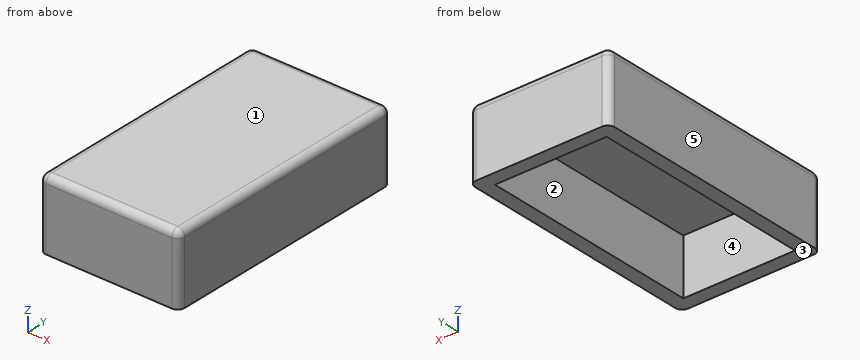
Autodesk Inventor part; units mm, degrees
ref_plane "YZ Plane" through (0, 0, 0) normal (1, 0, 0) x (0, 1, 0)
ref_plane "XZ Plane" through (0, 0, 0) normal (0, 1, 0) x (-1, 0, 0)
ref_plane "XY Plane" through (0, 0, 0) normal (0, 0, 1) x (1, 0, 0)
sketch "Sketch1" plane through (0, 0, 0) normal (0, 0, 1) x (1, 0, 0)
  line L0 (-25.4, -50.8) -> (25.4, -50.8)
  line L1 (25.4, -50.8) -> (25.4, 50.8)
  line L2 (25.4, 50.8) -> (-25.4, 50.8)
  line L3 (-25.4, 50.8) -> (-25.4, -50.8)
  line L4 (-25.4, -50.8) -> (25.4, 50.8) construction
  line L5 (25.4, -50.8) -> (-25.4, 50.8) construction
  point P0 (0, 0)
  dimension "d0" = 50.8
  dimension "d1" = 101.6
extrude "Extrusion1" add sketch "Sketch1" along normal blind 6.35
sketch "Sketch2" plane through (25.4, -50.8, 0) normal (1, 0, 0) x (0, 0, -1)
  line L0 (-6.35, 0) -> (-6.35, 101.6)
  line L1 (-6.35, 101.6) -> (0, 101.6)
  line L2 (0, 101.6) -> (0, 0)
  line L3 (0, 0) -> (-6.35, 0)
  line L4 (-6.35, 0) -> (-6.35, 101.6)
  point P0 (0, 50.8)
extrude "Extrusion2" add sketch "Sketch2" along normal blind 6.35
sketch "Sketch3" plane through (-25.4, -50.8, 0) normal (-1, 0, 0) x (0, 0, 1)
  point P0 (0, 50.8)
sketch "Sketch4" plane through (-25.4, -50.8, 0) normal (-1, 0, 0) x (0, 0, 1)
  line L0 (6.35, 101.6) -> (6.35, 0)
  line L1 (0, 0) -> (6.35, 0)
  line L2 (6.35, 101.6) -> (0, 101.6)
  line L3 (0, 101.6) -> (0, 0)
  line L4 (0, 0) -> (6.35, 0)
  line L5 (6.35, 0) -> (6.35, 101.6)
  point P0 (0, 50.8)
extrude "Extrusion3" add sketch "Sketch4" along normal blind 6.35
sketch "Sketch5" plane through (31.75, -50.8, 0) normal (0, -1, 0) x (1, 0, 0)
  line L0 (-63.5, 0) -> (-63.5, 6.35)
  line L1 (0, 6.35) -> (0, 0)
  line L2 (-63.5, 0) -> (0, 0)
  line L3 (0, 0) -> (0, 6.35)
  line L4 (0, 6.35) -> (-63.5, 6.35)
  line L5 (-63.5, 6.35) -> (-63.5, 0)
  point P0 (-31.75, 0)
extrude "Extrusion4" add sketch "Sketch5" along normal blind 6.35
sketch "Sketch6" plane through (31.75, 50.8, 6.35) normal (0, 1, 0) x (1, 0, 0)
  line L0 (-63.5, 0) -> (0, 0)
  line L1 (-63.5, 6.35) -> (0, 6.35)
  line L2 (-63.5, 0) -> (0, 0)
  line L3 (0, 0) -> (0, 6.35)
  line L4 (0, 6.35) -> (-63.5, 6.35)
  line L5 (-63.5, 6.35) -> (-63.5, 0)
  point P0 (-31.75, 6.35)
extrude "Extrusion5" add sketch "Sketch6" along normal blind 6.35
sketch "Sketch7" plane through (0, 0, 0) normal (0, 0, -1) x (-1, 0, 0)
  line L0 (31.75, -57.15) -> (31.75, 57.15)
  line L1 (31.75, -57.15) -> (25.4, -57.15)
  line L2 (25.4, -57.15) -> (25.4, 57.15)
  line L3 (25.4, 57.15) -> (31.75, 57.15)
  line L4 (31.75, 57.15) -> (31.75, -57.15)
  line L5 (-31.75, -57.15) -> (-25.4, -57.15)
  line L6 (-25.4, -57.15) -> (-25.4, 57.15)
  line L7 (-25.4, 57.15) -> (-31.75, 57.15)
  line L8 (-31.75, 57.15) -> (-31.75, -57.15)
  line L9 (25.4, -57.15) -> (-25.4, -57.15)
  line L10 (-25.4, -57.15) -> (-25.4, -50.8)
  line L11 (-25.4, -50.8) -> (25.4, -50.8)
  line L12 (25.4, -50.8) -> (25.4, -57.15)
  line L13 (25.4, 57.15) -> (-25.4, 57.15)
  line L14 (-25.4, 57.15) -> (-25.4, 50.8)
  line L15 (-25.4, 50.8) -> (25.4, 50.8)
  line L16 (25.4, 50.8) -> (25.4, 57.15)
  point P0 (0, 0)
  dimension "d12" = 6.35
  dimension "d13" = 114.3
  dimension "d14" = 6.35
  dimension "d15" = 114.3
  dimension "d16" = 50.8
  dimension "d17" = 6.35
  dimension "d18" = 6.35
  dimension "d19" = 50.8
extrude "Extrusion6" add sketch "Sketch7" along normal blind 25.4 contours L5 L8 L7 L6
sketch "Sketch8" plane through (25.4, -57.15, 0) normal (-1, 0, 0) x (0, 0, 1)
  line L0 (6.35, 0) -> (-25.4, 0)
  line L1 (-25.4, 0) -> (0, 0)
  line L2 (0, 0) -> (0, 6.35)
  line L3 (0, 6.35) -> (-25.4, 6.35)
  line L4 (-25.4, 6.35) -> (-25.4, 0)
  point P0 (0, 57.15)
  dimension "d22" = 25.4
  dimension "d23" = 6.35
extrude "Extrusion7" add sketch "Sketch8" along normal blind 57.15
sketch "Sketch9" plane through (25.4, 57.15, -25.4) normal (-1, 0, 0) x (0, 0, 1)
  line L0 (0, 0) -> (0, -114.3)
  line L1 (0, 0) -> (25.4, 0)
  line L2 (25.4, 0) -> (25.4, -6.35)
  line L3 (25.4, -6.35) -> (0, -6.35)
  line L4 (0, -6.35) -> (0, 0)
  point P0 (25.4, -57.15)
  dimension "d26" = 25.4
  dimension "d27" = 6.35
extrude "Extrusion8" add sketch "Sketch9" along normal blind 57.15
sketch "Sketch10" plane through (25.4, -50.8, 0) normal (0, 1, 0) x (1, 0, 0)
  line L0 (0, 25.4) -> (-57.15, 25.4)
  line L1 (-57.15, 25.4) -> (-50.8, 25.4)
  line L2 (-50.8, 25.4) -> (-50.8, 0)
  line L3 (-50.8, 0) -> (-57.15, 0)
  line L4 (-57.15, 0) -> (-57.15, 25.4)
  point P0 (-25.4, 0)
  dimension "d30" = 6.35
  dimension "d31" = 25.4
extrude "Extrusion9" add sketch "Sketch10" along normal blind 101.6
fillet "Fillet1" radius 3.175 1 edges at (0, -57.15, 6.35)
fillet "Fillet2" radius 3.175 3 edges at (-31.75, 1.5875, 6.35) (-31.75, -56.2201, 5.4201) (-31.75, -57.15, -11.1125)
fillet "Fillet3" radius 3.175 3 edges at (1.5875, 57.15, 6.35) (-30.8201, 57.15, 5.4201) (-31.75, 57.15, -11.1125)
fillet "Fillet4" radius 3.175 5 edges at (31.75, 0, 6.35) (31.75, 56.2201, 5.4201) (31.75, 57.15, -11.1125) (31.75, -56.2201, 5.4201) (31.75, -57.15, -11.1125)
properties part number "Table foot"
Geometry: final body of the model. Coordinates: model frame, mm. Face numbers are marked on the shaded views. A direction names the side the tool comes from. Coordinates: 2 decimals unless noted, no trailing zeros. Order: outer loops, then holes, each group sorted by start corner. A loop starts at its lowest first (then second) coordinate and runs counter-clockwise, first axis right, second up.
(1) Access query for the marked faces 1 and 2. Directions: +Z, -Z, +X, -X, +Y, -Y. A direction counts if a zero-diameter tool reaches every point of the face in a straight line with its end or side. Return the directions, or none.
(2) Draft query along X for the marked faces 3, 4 and 5. Return one class per face: pulls with the +X half, pulls with the -X half, needs draft (parallel to the pull), parting line crosses it, or undercut.
(3) First-contact query: pin 1 (1.5 mm diameter, centred on x = -11, y = 31.5, fed in from -Z). Flat tip, straight axial feed; report the tip coordinate or a pass-through.
(4) Section query C-C (x = 5.5). Return the cut outline in (y, z) (3 decimals), plus the area to 3 significant figures.
(5) Material intervals for probe 1 along Y at (x, z) = (-21.5, -17.5); probe 2 along X at (y, z) = (48, -19); probe 3 along Z at (x, y) = (5, -36), sorted ascending.
(6) Section query B-B (y = 30.5). Return the cut outline in (x, z) (3 decimals).
(7) Section query A-A (z = -17). Return the cut outline in (x, y) (3 decimals), plus the area to 3 significant figures.
Solution:
1. face 1: +Z, +X, -X, +Y, -Y
1. face 2: -Z
2. face 3: needs draft
2. face 4: undercut
2. face 5: pulls with the -X half
3. pin 1: stops at z = 0
4. outline: (-57.15, -25.4) - (-50.8, -25.4) - (-50.8, 0) - (50.8, 0) - (50.8, -25.4) - (57.15, -25.4) - (57.15, 3.175) arc R3.175 ccw to (53.975, 6.35) - (-53.975, 6.35) arc R3.175 ccw to (-57.15, 3.175) - close
4. area: 1,040 mm2
5. probe 1: y = -57.15 to -50.8, 50.8 to 57.15
5. probe 2: x = -31.75 to -25.4, 25.4 to 31.75
5. probe 3: z = 0 to 6.35
6. outline: (-31.75, -25.4) - (-25.4, -25.4) - (-25.4, 0) - (25.4, 0) - (25.4, -25.4) - (31.75, -25.4) - (31.75, 3.175) arc R3.175 ccw to (28.575, 6.35) - (-28.575, 6.35) arc R3.175 ccw to (-31.75, 3.175) - close
7. outline: (-31.75, -53.975) arc R3.175 ccw to (-28.575, -57.15) - (28.575, -57.15) arc R3.175 ccw to (31.75, -53.975) - (31.75, 53.975) arc R3.175 ccw to (28.575, 57.15) - (-28.575, 57.15) arc R3.175 ccw to (-31.75, 53.975) - close; hole (-25.4, -50.8) - (25.4, -50.8) - (25.4, 50.8) - (-25.4, 50.8) - close
7. area: 2,090 mm2
